Check sheet for the modelled part. Datum: model origin and axes. Units: mm. A direction names the side the tool comes from. Give positions to 0.01 mm unless a question says otherwise; leave off trailing zeros. Write each loop counter-clockwise with the first axis right and the second up, starting at its lowest first coordinate (ties: lowest second). Pieces come first, ordered by that corner, then holes. Notation, with made-up numbers: (-9, 62.25) -> (30, 62.25) arc R33 ccw to (30, 93.25) -> close; hole circle Ø3 at (44, 44). An arc over 180 degrees is marked (long way). Return JSON: item names as keys, results as strings.
from build123d import *

# Parameters (mm, degrees)
F0_W     = 110
F0_H     = 50
F1_DEPTH = 5
F2_W     = 6.5
F2_H     = 6.5
F3_DEPTH = 5


with BuildPart() as f1:
    # F0 (on Top) → F1 (new body)
    with BuildSketch(Plane.XY):
        with Locations((2.586676, 5.525514)):
            Rectangle(F0_W, F0_H)
    extrude(amount=F1_DEPTH)

    # F2 (on face) → F3 (join)
    with BuildSketch(Plane.XY.offset(5)):
        with Locations((-44.919127, 23.786242)):
            Rectangle(F2_W, F2_H)
        with Locations((-34.35, 23.85)):
            Rectangle(F2_W, F2_H)
        with Locations((-23.780873, 23.913758)):
            Rectangle(F2_W, F2_H)
        with Locations((-13.211747, 23.977516)):
            Rectangle(F2_W, F2_H)
        with Locations((-2.64262, 24.041274)):
            Rectangle(F2_W, F2_H)
        with Locations((7.926506, 24.105032)):
            Rectangle(F2_W, F2_H)
        with Locations((18.495633, 24.16879)):
            Rectangle(F2_W, F2_H)
        with Locations((29.06476, 24.232548)):
            Rectangle(F2_W, F2_H)
        with Locations((39.633886, 24.296306)):
            Rectangle(F2_W, F2_H)
        with Locations((50.203013, 24.360064)):
            Rectangle(F2_W, F2_H)
        with Locations((-44.918754, 12.968144)):
            Rectangle(F2_W, F2_H)
        with Locations((-34.428743, 12.95)):
            Rectangle(F2_W, F2_H)
        with Locations((-23.938732, 12.931856)):
            Rectangle(F2_W, F2_H)
        with Locations((-13.44872, 12.913711)):
            Rectangle(F2_W, F2_H)
        with Locations((-2.958709, 12.895567)):
            Rectangle(F2_W, F2_H)
        with Locations((7.531302, 12.877423)):
            Rectangle(F2_W, F2_H)
        with Locations((18.021314, 12.859278)):
            Rectangle(F2_W, F2_H)
        with Locations((28.511325, 12.841134)):
            Rectangle(F2_W, F2_H)
        with Locations((39.001336, 12.82299)):
            Rectangle(F2_W, F2_H)
        with Locations((49.491347, 12.804845)):
            Rectangle(F2_W, F2_H)
        with Locations((-44.918754, 2.76096)):
            Rectangle(F2_W, F2_H)
        with Locations((-34.55, 2.95)):
            Rectangle(F2_W, F2_H)
        with Locations((-24.181246, 3.13904)):
            Rectangle(F2_W, F2_H)
        with Locations((-13.812492, 3.32808)):
            Rectangle(F2_W, F2_H)
        with Locations((-3.443738, 3.51712)):
            Rectangle(F2_W, F2_H)
        with Locations((6.925016, 3.70616)):
            Rectangle(F2_W, F2_H)
        with Locations((17.29377, 3.8952)):
            Rectangle(F2_W, F2_H)
        with Locations((27.662524, 4.08424)):
            Rectangle(F2_W, F2_H)
        with Locations((38.031278, 4.27328)):
            Rectangle(F2_W, F2_H)
        with Locations((48.400033, 4.462319)):
            Rectangle(F2_W, F2_H)
    extrude(amount=F3_DEPTH)


solid = f1.part
(1) Thickness scan on L1, parallel to Y at x = 38.5, z = 6; L2, parallel to Y at x = -33, z = 9; L3, parallel to Y at x = 42, z = 6. Record the ranges inside material, lowest first.
Reply:
{"L1": "1.02 to 7.52, 9.57 to 16.07, 21.05 to 27.55", "L2": "-0.3 to 6.2, 9.7 to 16.2, 20.6 to 27.1", "L3": "9.57 to 16.07, 21.05 to 27.55"}
(2) Release check for a two-part mould opening along X. For faces 1 (the flat face through (14.044, 4, 7)), 2 (the flat face through (51.65, 4, 7)), 3 (the flat face through (48, 5, 10)), 4 (the flat face through (30.913, 4, 7)) record: pulls with the +X half, pulls with the -X half, needs draft (parallel to the pull), parting line crosses it, or undercut.
Reply:
{"face 1": "undercut", "face 2": "pulls with the +X half", "face 3": "needs draft", "face 4": "undercut"}
(3) Set-up check for faces 5 (the flat face through (-0.194, 3, 7)), 6 (the flat face through (4.281, 13, 7)): record each of +Z, -Z, +X, -X, +Y, -Y from which the full face is reachable in a straight line by a thin tool's end or side.
Reply:
{"face 5": "+Z, -Y", "face 6": "+Z, +Y"}
(4) Cross-section at C-C on y = -15.5. Enter the section's corners in (x, z), then the cut area to 3 significant figures.
Reply:
{"outline": "(-52.41, 0) -> (57.59, 0) -> (57.59, 5) -> (-52.41, 5) -> close", "area": "550 mm^2"}
(5) Cross-section at B-B on z = 8.25. State how many separate pieces and enclosed holes the cut face has, then the cut area to 3 significant figures.
Reply:
{"separate pieces": "30", "enclosed holes": "0", "area": "1,270 mm^2"}
(6) Depth check by flat-ended pin: pin 1 Ø1.5 at (x, z) = (-23, 7) entering from -Y; pin 2 Ø5.5 at (x, z) = (19.5, 8) entering from +Y; pin 3 Ø4 at (y, z) = (25, 7.5) entering from +X. Enter the tip coordinate at first touch or a pass-through.
Reply:
{"pin 1": "y = -0.11", "pin 2": "y = 27.42", "pin 3": "x = 53.45"}
(7) Cross-section at A-A on x = 48.5. Enter the section's corners in (y, z).
Reply:
{"outline": "(-19.47, 0) -> (30.53, 0) -> (30.53, 5) -> (27.61, 5) -> (27.61, 10) -> (21.11, 10) -> (21.11, 5) -> (16.05, 5) -> (16.05, 10) -> (9.55, 10) -> (9.55, 5) -> (7.71, 5) -> (7.71, 10) -> (1.21, 10) -> (1.21, 5) -> (-19.47, 5) -> close"}
